```python
from build123d import *

# Parameters (mm, degrees)
F1_DEPTH = 40
F3_DEPTH = 20
F4_W     = 10
F4_H     = 20
F5_DEPTH = 20


with BuildPart() as f1:
    # F0 (on Front) → F1 (new body)
    with BuildSketch(Plane.XZ):
        Polygon((31.704547, 10.600731), (1.704547, 10.600731), (-18.295453, 10.600731), (-18.295453, -9.399269), (31.704547, -9.399269), align=None)
    extrude(amount=F1_DEPTH)

    # F2 (on face) → F3 (cut)
    with BuildSketch(Plane.XZ.offset(40)):
        Polygon((-18.295453, 10.600731), (-18.295453, -9.399269), (0, 10.600731), align=None)
    extrude(amount=-F3_DEPTH, mode=Mode.SUBTRACT)

    # F4 (on face) → F5 (join)
    with BuildSketch(Plane.XY.offset(10.600731)):
        with Locations((15, -20)):
            Rectangle(F4_W, F4_H)
    extrude(amount=F5_DEPTH)


solid = f1.part
```
The listing builds one solid part. Answer for the finished solid, in the listing's coordinates (mm). A direction names the side the tool comes from. Give positions to 0.01 mm unless a question says otherwise; leave off trailing zeros. Write each loop counter-clockwise with the first axis right and the second up, starting at its lowest first coordinate (ties: lowest second). Pieces come first, ordered by that corner, then holes. Notation, with made-up numbers: (-13.5, -27) - (30.5, -27) arc R18 ccw to (30.5, 3) - close; hole circle Ø9 at (-12, 51). An arc over 180 degrees is marked (long way). Use one line per item in the form item = value. Start each with the question number.
1) Find section B-B on x = 17. Determine the outline of the cut face in (y, z).
2) Find section C-C on z = 20.5. Determine the outline of the cut face in (x, y), plus the area to 3 significant figures.
3) Flat-ended cylindrical pins translate along their axes: pin 1 Ø5 at (x, z) = (13, 23.5) entering from +Y; pin 2 Ø10 at (y, z) = (-23, 17) entering from +X; pin 3 Ø8 at (y, z) = (-29.5, 15) entering from -X. Find the tip coordinate at first contact, or state that the pin passes through.
4) A tool of negligible diameter and unlimited length cuts with its end or side. For faces 1 (the face through (10, -20, 20)), 2 (the face through (15, -10, 20)), 3 (the face through (-11, -20, 3)), 4 (the face through (20, -20, 20)), from which of +Z, -Z, +X, -X, +Y, -Y can it reach the whole face along a straight path? Write none if from no direction.
5) Consider line 1 along Z through (x, y) = (-16, -9.5); line 2 along X through (y, z) = (-24, 21); line 3 along Y through (x, z) = (-14.5, -1). Determine where each line is inside the solid, lowest interval first. Write a range as from..to.
6) Find section D-D on x = -1. Determine the outline of the cut face in (y, z).
7) Find section A-A on y = -15.5. Determine the outline of the cut face in (x, z).
Geometry results:
q1.outline = (-40, -9.4) - (0, -9.4) - (0, 10.6) - (-10, 10.6) - (-10, 30.6) - (-30, 30.6) - (-30, 10.6) - (-40, 10.6) - close
q2.outline = (10, -30) - (20, -30) - (20, -10) - (10, -10) - close
q2.area = 200 mm2
q3.pin_1 = -10
q3.pin_2 = 20
q3.pin_3 = 10
q4.face_1 = +Z, -X, +Y, -Y
q4.face_2 = +Z, +X, -X, +Y
q4.face_3 = +Z, -X, -Y
q4.face_4 = +Z, +X, +Y, -Y
q5.line_1 = -9.4..10.6
q5.line_2 = 10..20
q5.line_3 = -20..0
q6.outline = (-40, -9.4) - (0, -9.4) - (0, 10.6) - (-20, 10.6) - (-20, 9.51) - (-40, 9.51) - close
q7.outline = (-18.3, -9.4) - (31.7, -9.4) - (31.7, 10.6) - (20, 10.6) - (20, 30.6) - (10, 30.6) - (10, 10.6) - (-18.3, 10.6) - close
